```python
from build123d import *

# Parameters (mm, degrees)
SKETCH1_W           = 1.5875
SKETCH1_H           = 19.05
BOSS_EXTRUDE1_DEPTH = 1.5875


with BuildPart() as part:
    # Sketch1 → Boss-Extrude1 (new body)
    with BuildSketch(Plane(origin=(0, 0, 0), x_dir=(1, 0, 0), z_dir=(0, 1, 0))):
        with BuildLine():
            Line((11.1125, 27.788669701), (11.1125, -30.963669701))
            ThreePointArc((11.1125, -30.963669701), (0, -19.851169701), (-11.1125, -30.963669701))
            Line((-11.1125, -30.963669701), (-11.1125, 27.788669701))
            ThreePointArc((-11.1125, 27.788669701), (0, 16.676169701), (11.1125, 27.788669701))
        make_face()
        with Locations((11.90625, -1.5875)):
            Rectangle(SKETCH1_W, SKETCH1_H)
        with Locations((-11.90625, -1.5875)):
            Rectangle(SKETCH1_W, SKETCH1_H)
    extrude(amount=BOSS_EXTRUDE1_DEPTH)


solid = part.part
```
The model under review builds one solid part; all positions refer to its coordinate system, in mm. A direction names the side the tool comes from. Give positions to 0.01 mm unless a question says otherwise; leave off trailing zeros. Write each loop counter-clockwise with the first axis right and the second up, starting at its lowest first coordinate (ties: lowest second). Pieces come first, ordered by that corner, then holes.
(1) For P1, Ø0.8, axis at y = 0.5, z = -22.5, coming from the +X side; P2, Ø0.5, axis at y = 1, z = -19, coming from the -X side; P3, Ø0.8, axis at x = 12.5, y = 1, coming from the -Z side, all flat-tipped, find the tip position at first contact; note any pin that passes through.
(2) Tool access review of faces 1 (the flat face through (12, 1, -7.938)), 2 (the flat face through (-12, 1, 11.112)), 3 (the flat face through (-12, 1, -7.938)), 4 (the flat face through (11.112, 1, 21)): name each direction out of +Z, -Z, +X, -X, +Y, -Y from which nothing blocks a thin tool from reaching the whole face with its end or side.
(3) Consider section B-B, the plane y = 0.3. Give the boundary of the cut face in (x, z) (1 decimal).
(4) The part is to be moulded in two halves that separate along X. For faces 5 (the cylindrical face through (-0.24, 0.78, -16.68)), 6 (the flat face through (0, 0, 1)), 7 (the flat face through (-11.112, 1, 21)), say which applies: released by +X, released by -X, zero draft, split by the parting line, or undercut.
(5) Consider section A-A, the plane z = 26. Give the boundary of the cut face in (x, y), and give its area (3 significant figures).
(6) To check wall thickness, follow L1, parallel to X at y = 0.8, z = 23; L2, parallel to Z at x = 0.25, y = 0.15; L3, parallel to X at y = 0.3, z = 17. State the ranges of each line that lie inside material, in increasing order.
(7) Consider section D-D, the plane z = -9.5. Give the boundary of the cut face in (x, y).
(8) Consider section C-C, the plane x = 0. Give the boundary of the cut face in (y, z), and give its area (3 significant figures).
Returned:
1. P1: stops at x = 11.11
1. P2: stops at x = -11.11
1. P3: stops at z = -7.94
2. face 1: -Z, +X, +Y, -Y
2. face 2: +Z, -X, +Y, -Y
2. face 3: -Z, -X, +Y, -Y
2. face 4: +Z, +X, +Y, -Y
3. outline: (-12.7, -7.9) - (-11.1, -7.9) - (-11.1, -27.8) arc R11.1 cw to (11.1, -27.8) - (11.1, -7.9) - (12.7, -7.9) - (12.7, 11.1) - (11.1, 11.1) - (11.1, 31) arc R11.1 cw to (-11.1, 31) - (-11.1, 11.1) - (-12.7, 11.1) - close
4. face 5: undercut
4. face 6: zero draft
4. face 7: released by -X
5. outline: (-11.11, 0) - (-9.94, 0) - (-9.94, 1.59) - (-11.11, 1.59) - close; (9.94, 0) - (11.11, 0) - (11.11, 1.59) - (9.94, 1.59) - close
5. area: 3.72 mm2
6. L1: x = -11.11 to -7.75, 7.75 to 11.11
6. L2: z = -16.68 to 19.85
6. L3: x = -11.11 to 11.11
7. outline: (-11.11, 0) - (11.11, 0) - (11.11, 1.59) - (-11.11, 1.59) - close
8. outline: (0, -16.68) - (1.59, -16.68) - (1.59, 19.85) - (0, 19.85) - close
8. area: 58.0 mm2
